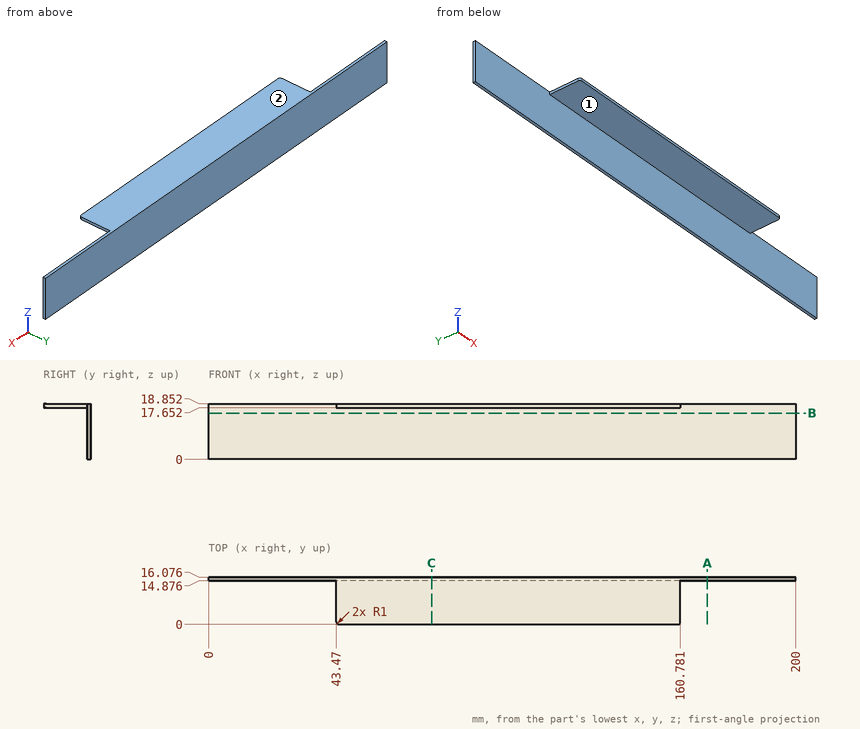
For this review, use the dimensioned drawing (mm, ordinates from the lowest corner) and the shaded views. A direction names the side the tool comes from. Give positions to 0.01 mm unless a question says otherwise; leave off trailing zeros. Order: outer loops, then holes, each group sorted by start corner. A loop starts at its lowest first (then second) coordinate and runs counter-clockwise, first axis right, second up. Notation, with made-up numbers: (-23, -8) - (26, -8) arc R18 cw to (26, 22) - close; hole circle Ø5 at (4, 26). An arc over 180 degrees is marked (long way). Use CSV: the item, a comma, the result in double quotes. Start each with the question number.
Q1. Machinability: for the marked faces 1 and 2, which of the approach directions +Z, -Z, +X, -X, +Y, -Y give a long, thin tool a straight path to every point of the face, cutting with its end or side? Answer none if there is none.
Q2. For line 1 (Z direction, x = 43.5, y = 14); line 2 (Y direction, x = 118.5, z = 8.75), list the stretches that pass through material, from the lowest coordinate up.
Q3. For P1, Ø3, axis at x = 147, y = 5.5, coming from the -Z side; P2, Ø0.6, axis at y = 7, z = 18.5, coming from the +X side; P3, Ø6, axis at x = 33, y = 11, coming from the -Z side; P4, Ø4, axis at x = 93.5, z = 6.5, coming from the -Y side, all flat-tipped, find the tip position at first contact; note any pin that passes through.
Q4. Take a section at C-C (x = 76). State the section outline as (y, z) points.
Q5. Take a section at B-B (z = 15.75). State the section outline as (x, y) points, and give its area (3 significant figures).
Q6. Take a section at A-A (x = 170). State the section outline as (y, z) points.
Calculated:
1,face 1,"-Z, +X, -X, -Y"
1,face 2,"+Z, +X, -X, +Y, -Y"
2,line 1,"z = 17.65 to 18.85"
2,line 2,"y = 14.88 to 16.08"
3,P1,"stops at z = 17.65"
3,P2,"stops at x = 160.78"
3,P3,"passes through"
3,P4,"stops at y = 14.88"
4,outline,"(0, 17.65) - (14.88, 17.65) - (14.88, 0) - (16.08, 0) - (16.08, 18.85) - (0, 18.85) - close"
5,outline,"(0, 14.88) - (200, 14.88) - (200, 16.08) - (0, 16.08) - close"
5,area,"240 mm²"
6,outline,"(14.88, 0) - (16.08, 0) - (16.08, 18.85) - (14.88, 18.85) - close"
